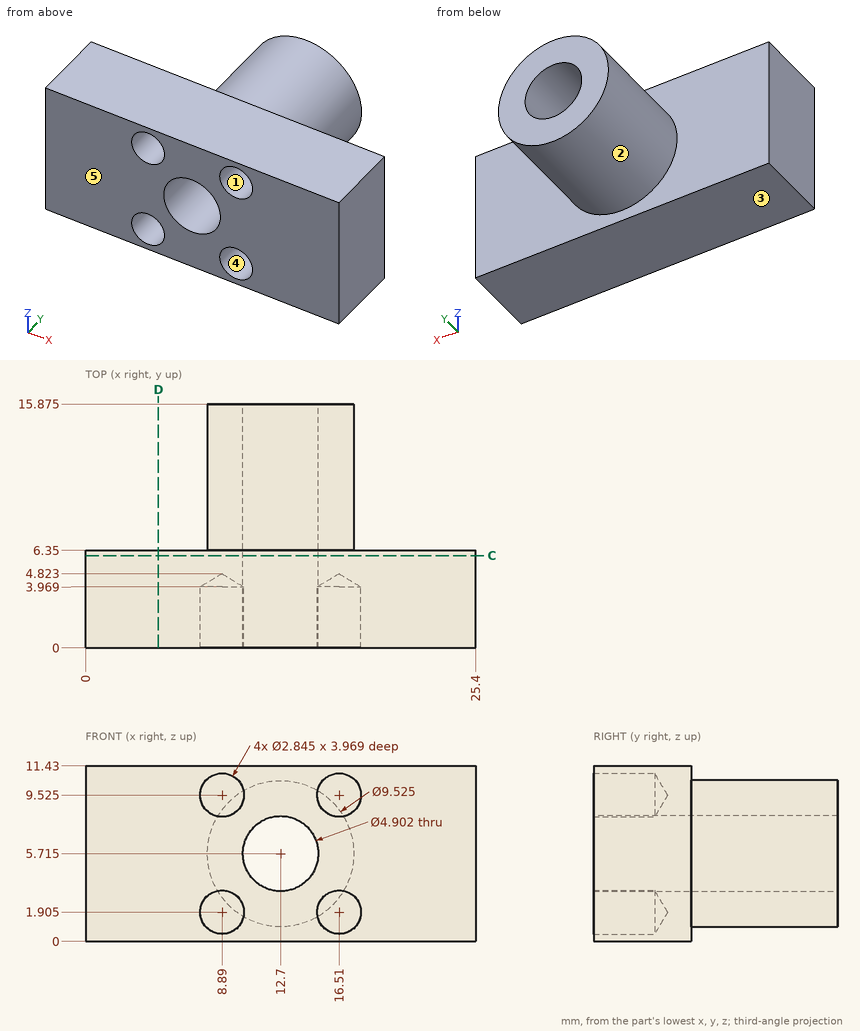
Answer from the drawing. Dimensions are ordinates in mm from the lowest x, y and z of the part. A direction names the side the tool comes from. Give positions to 0.01 mm unless a question says otherwise; leave off trailing zeros. Loops run counter-clockwise (first coordinate to the right, second up) from the corner with the lowest first, then second, coordinate; pieces in that order, holes last.
Item 1: Find the intervals of material crossed by line 1 along Z through (x, y) = (16.51, 1.25); line 2 along Y through (x, z) = (7, 2); line 3 along X through (y, z) = (2.5, 7.25), in increasing order.
Item 2: For the marked faces 4 and 5, determine the directions among +Z, -Z, +X, -X, +Y, -Y from which every point of the face is accessible in a straight line to the end or side of a thin tool.
Item 3: The mould has two halves that part along Z. Classify the marked faces 1, 2 and 3: released by +Z, released by -Z, zero draft, split by the parting line, or undercut.
Item 4: Each of these flat-tipped pins is pushed along its axis until it touches: pin 1 Ø1.5 at (x, z) = (5, 3.5) entering from +Y; pin 2 Ø2.5 at (x, z) = (8.89, 1.905) entering from +Y (3 decimals); pin 3 Ø2.5 at (x, z) = (16.51, 9.525) entering from -Y; pin 4 Ø2 at (y, z) = (13.5, 5) entering from +X. Where does it stop, or does it pass through?
Item 5: The part is cut by section C-C (y = 6). Write down the section's boundary in (x, z) (1 decimal).
Item 6: The part is cut by section D-D (x = 4.75). Write down the section's boundary in (y, z), and give its area (3 significant figures).
Taken from the geometry:
1. line 1: z = 0 to 0.48, 3.33 to 8.1, 10.95 to 11.43
1. line 2: y = 0 to 6.35
1. line 3: x = 0 to 10.79, 14.61 to 25.4
2. face 4: -Y
2. face 5: +Z, -Z, +X, -X, -Y
3. face 1: undercut
3. face 2: split by the parting line
3. face 3: released by -Z
4. pin 1: stops at y = 6.35
4. pin 2: stops at y = 15.875
4. pin 3: stops at y = 4.07
4. pin 4: stops at x = 17.46
5. outline: (0, 0) - (25.4, 0) - (25.4, 11.4) - (0, 11.4) - close; hole circle Ø4.9 at (12.7, 5.7)
6. outline: (0, 0) - (6.35, 0) - (6.35, 11.43) - (0, 11.43) - close
6. area: 72.6 mm2
